Build history of the part. All positions in model axes, mm. A direction names the side the tool comes from. Coordinates: 2 decimals unless noted, no trailing zeros. Order: outer loops, then holes, each group sorted by start corner. A loop starts at its lowest first (then second) coordinate and runs counter-clockwise, first axis right, second up. Notation, with made-up numbers: (60.5, 50) - (91.5, 50) arc R12 ccw to (91.5, 60) - close; hole circle Ø3 at (69.5, 46). An arc over 180 degrees is marked (long way). One line per item, written item: value.
Autodesk Inventor part; units mm, degrees
ref_plane "YZ Plane" through (0, 0, 0) normal (1, 0, 0) x (0, 1, 0)
ref_plane "XZ Plane" through (0, 0, 0) normal (0, 1, 0) x (-1, 0, 0)
ref_plane "XY Plane" through (0, 0, 0) normal (0, 0, 1) x (1, 0, 0)
sketch "Sketch1" plane through (0, 0, 0) normal (0, 1, 0) x (-1, 0, 0)
  line L0 (0, -471.17) -> (0, 471.17)
  line L1 (471.17, 0) -> (-471.17, 0)
  line L2 (-333.375, 333.375) -> (333.375, 333.375)
  line L3 (333.375, 333.375) -> (333.375, -333.375)
  line L4 (333.375, -333.375) -> (-333.375, -333.375)
  line L5 (-333.375, -333.375) -> (-333.375, 333.375)
  line L6 (-298.45, 298.45) -> (298.45, 298.45)
  line L7 (298.45, 298.45) -> (298.45, -298.45)
  line L8 (298.45, -298.45) -> (-298.45, -298.45)
  line L9 (-298.45, -298.45) -> (-298.45, 298.45)
  line L10 (-336.55, 336.55) -> (336.55, 336.55)
  line L11 (336.55, 336.55) -> (336.55, -336.55)
  line L12 (336.55, -336.55) -> (-336.55, -336.55)
  line L13 (-336.55, -336.55) -> (-336.55, 336.55)
  point P0 (0, 0)
  dimension "d0" = 666.75
  dimension "d1" = 666.75
  dimension "d4" = 3.175
  dimension "d5" = 3.175
  dimension "d50" = 38.1
  dimension "d51" = 38.1
extrude "Extrusion1" add sketch "Sketch1" against normal blind 3.175 contours L12 L13 L1 L5 L4 L0 | L0 L4 L3 L1 L11 L12 | L4 L5 L1 L9 L8 L0 | L0 L8 L7 L1 L3 L4 | L1 L3 L2 L0 L10 L11 | L13 L10 L0 L2 L5 L1 | L1 L7 L6 L0 L2 L3 | L5 L2 L0 L6 L9 L1
extrude "Extrusion2" add sketch "Sketch1" along normal blind 34.925 contours L12 L13 L1 L5 L4 L0 | L0 L4 L3 L1 L11 L12 | L1 L3 L2 L0 L10 L11 | L13 L10 L0 L2 L5 L1
sketch "Sketch2" plane through (0, 34.925, 0) normal (0, 1, 0) x (1, 0, 0)
  line L0 (336.55, -336.55) -> (336.55, 336.55)
  line L1 (336.55, 336.55) -> (-336.55, 336.55)
  line L2 (301.625, 336.55) -> (336.55, 336.55)
  line L3 (339.725, 339.725) -> (301.625, 339.725)
  line L4 (301.625, 339.725) -> (301.625, 336.55)
  line L5 (339.725, 339.725) -> (339.725, 301.625)
  line L6 (339.725, 301.625) -> (336.55, 301.625)
  line L7 (336.55, 301.625) -> (336.55, 336.55)
  point P0 (0, 0)
  dimension "d10" = 3.175
  dimension "d15" = 3.175
  dimension "d52" = 38.1
  dimension "d53" = 38.1
extrude "Extrusion3" add sketch "Sketch2" against normal blind 601.6625
sketch "Sketch4" plane through (336.55, -3.175, 336.55) normal (1, 0, 0) x (0, 0, -1)
  line L0 (673.1, 0) -> (0, 0)
  line L1 (377.7476, 24.6957) -> (350.8068, -2.2451)
  line L2 (350.8068, -2.2451) -> (638.175, -289.6133)
  line L3 (638.175, -289.6133) -> (638.175, -235.7317)
  line L4 (638.175, -235.7317) -> (377.7476, 24.6957)
  line L5 (638.175, 38.1) -> (638.175, -563.5625)
  line L6 (676.275, -563.5625) -> (638.175, -563.5625)
  line L7 (353.0519, 0) -> (638.175, -285.1231)
  line L8 (353.0519, 0) -> (350.8068, -2.2451)
  line L9 (350.8068, -2.2451) -> (638.175, -289.6133)
  line L10 (638.175, -289.6133) -> (638.175, -285.1231)
  line L11 (638.175, -285.1231) -> (353.0519, 0)
  point P0 (336.55, 3.175)
  point P1 (676.275, -339.725)
  dimension "d23" = 38.1
  dimension "d28" = 3.175
  dimension "d47" = 45
  dimension "d49" = 406.4
extrude "Extrusion5" add sketch "Sketch4" against normal blind 34.925 contours L7 L3 L2 L1
extrude "Extrusion6" add sketch "Sketch4" along normal blind 3.175 contours L4 L3 L7 L0 | L0 L1 L4 | L7 L3 L2 L1
sketch "Sketch5" plane through (339.725, 34.925, -339.725) normal (0, 0, -1) x (-1, 0, 0)
  line L0 (38.1, 0) -> (38.1, -601.6625)
  line L1 (676.275, -38.1) -> (38.1, -38.1)
  line L2 (676.275, 0) -> (676.275, -38.1)
  line L3 (38.1, 0) -> (676.275, 0)
  line L4 (38.1, -327.7133) -> (325.4682, -40.3451)
  line L5 (325.4682, -40.3451) -> (298.5274, -13.4043)
  line L6 (298.5274, -13.4043) -> (38.1, -273.8317)
  line L7 (38.1, -273.8317) -> (38.1, -327.7133)
  line L8 (323.2231, -38.1) -> (38.1, -323.2231)
  line L9 (38.1, 0) -> (38.1, -38.1)
  point P0 (0, -381)
  point P1 (339.725, -34.925)
  dimension "d33" = 38.1
  dimension "d35" = 3.175
  dimension "d45" = 45
  dimension "d48" = 406.4
extrude "Extrusion7" add sketch "Sketch5" against normal blind 3.175 contours L6 L1 L8 L0 | L6 L5 L1 | L8 L5 L4 L0
extrude "Extrusion8" add sketch "Sketch5" against normal blind 38.1 contours L8 L5 L4 L0
mirror "Mirror1" about plane through (0, 0, 0) normal (0, 0, 1) of "Extrusion8", "Extrusion7", "Extrusion6", "Extrusion5", "Extrusion3"
mirror "Mirror2" about plane through (0, 0, 0) normal (1, 0, 0) of "Extrusion8", "Extrusion7", "Extrusion6", "Extrusion5", "Extrusion3", "Mirror1"
properties part number "Single_Burner_Stand"
1. 3-axis set-ups, long thin cutter, end or side, ignore diameter. For faces 4 (the face through (-259, -221, -336.55)), 5 (the face through (157, -147, 301.625)), 6 (the face through (333.375, 17, -5)): which of +Z, -Z, +X, -X, +Y, -Y reach the whole face in a straight line?
Values found:
face 4: none
face 5: -Y
face 6: +Y
2. Band-saw the part on B-B, the plane z = 278. Give the cut face in (x, y) (3 decimals), and give its area (3 significant figures).
Values found:
outline: (-339.725, -269.163) - (-301.625, -269.163) - (-301.625, -264.673) - (-336.55, -264.673) - (-336.55, -215.282) - (-339.725, -215.282) - close; (-336.55, -3.175) - (-298.45, -3.175) - (-298.45, 0) - (-333.375, 0) - (-333.375, 34.925) - (-336.55, 34.925) - close; (298.45, -3.175) - (336.55, -3.175) - (336.55, 34.925) - (333.375, 34.925) - (333.375, 0) - (298.45, 0) - close; (301.625, -269.163) - (339.725, -269.163) - (339.725, -215.282) - (336.55, -215.282) - (336.55, -264.673) - (301.625, -264.673) - close
area: 1,120 mm2
3. Flat gauge pins, fed straight in: P1, Ø11.5, axis at y = 24, z = 18, coming from the +X side; P2, Ø19, axis at y = 19, z = 23, coming from the -X side. Where does each tip first touch, or does it go through?
Values found:
P1: stops at x = 336.55
P2: stops at x = -336.55
4. Band-saw the part on C-C, the plane x = -54.5. Give the cut face in (y, z) (3 decimals).
Values found:
outline: (-45.663, -339.725) - (8.218, -339.725) - (8.218, -336.55) - (34.925, -336.55) - (34.925, -333.375) - (0, -333.375) - (0, -298.45) - (-3.175, -298.45) - (-3.175, -336.55) - (-41.173, -336.55) - (-41.173, -301.625) - (-45.663, -301.625) - close; (-45.663, 301.625) - (-41.173, 301.625) - (-41.173, 336.55) - (-3.175, 336.55) - (-3.175, 298.45) - (0, 298.45) - (0, 333.375) - (34.925, 333.375) - (34.925, 336.55) - (8.218, 336.55) - (8.218, 339.725) - (-45.663, 339.725) - close
5. Band-saw the part on A-A, the plane y = -336.5. Give the cut face in (x, z) (3 decimals), and give its area (3 significant figures).
Values found:
outline: (-339.725, -339.725) - (-301.625, -339.725) - (-301.625, -336.55) - (-336.55, -336.55) - (-336.55, -301.625) - (-339.725, -301.625) - close; (-339.725, 301.625) - (-336.55, 301.625) - (-336.55, 336.55) - (-301.625, 336.55) - (-301.625, 339.725) - (-339.725, 339.725) - close; (301.625, -339.725) - (339.725, -339.725) - (339.725, -301.625) - (336.55, -301.625) - (336.55, -336.55) - (301.625, -336.55) - close; (301.625, 336.55) - (336.55, 336.55) - (336.55, 301.625) - (339.725, 301.625) - (339.725, 339.725) - (301.625, 339.725) - close
area: 927 mm2
6. Probe line 1 along X through (y, z) = (-207.5, -231) (3 decimals); line 2 along X through (y, z) = (-157.5, -305) (3 decimals); line 3 along Y through (x, z) = (-308.5, -225) (3 decimals). List the from-to ranges inside material, lowest first.
Values found:
line 1: x = -339.725 to -336.55, 336.55 to 339.725
line 2: x = -339.725 to -336.55, -170.827 to -166.337, 166.337 to 170.827, 336.55 to 339.725
line 3: y = -216.163 to -211.673, -3.175 to 0
7. Two-plate mould, pull along X, no slides. Class faces 1 (the face through (5, 17, 333.375)), 2 (the face through (336.55, 16, -4)), 3 (the face through (320.942, -147.093, -155.929)): pulls with the +X half, pulls with the -X half, needs draft (parallel to the pull), parting line crosses it, or undercut.
Values found:
face 1: undercut
face 2: pulls with the +X half
face 3: needs draft
8. Band-saw the part on D-D, the plane y = -68. Count the separate pieces of the cut face and the enclosed holes in it, and give its area (3 significant figures).
Values found:
separate pieces: 12
enclosed holes: 0
area: 3,550 mm2
